Autodesk Inventor part; units mm, degrees
ref_plane "Work Plane1" through (0, 7.5, 0) normal (0, 1, 0) x (1, 0, 0)
ref_plane "YZ Plane" through (0, 0, 0) normal (1, 0, 0) x (0, 1, 0)
ref_plane "XZ Plane" through (0, 0, 0) normal (0, 1, 0) x (-1, 0, 0)
sketch "Sketch1" plane through (0, 0, 0) normal (0, 1, 0) x (-1, 0, 0)
  circle A0 centre (0, 0) radius 12.5
  dimension "d0" = 25
extrude "Extrusion1" add sketch "Sketch1" along normal blind 19 and the other way blind 15
sketch "Sketch2" plane through (0, 0, 0) normal (0, 0, 1) x (1, 0, 0)
  line L0 (-5.25, -15) -> (-5.25, -7.5)
  arc A0 (5.25, -7.5) -> (-5.25, -7.5) centre (0, -7.5) ccw
  line L1 (5.25, -7.5) -> (5.25, -15)
  line L2 (5.25, -15) -> (-5.25, -15)
  line L3 (-3.1, -15) -> (-3.1, -7.5)
  arc A1 (3.1, -7.5) -> (-3.1, -7.5) centre (0, -7.5) ccw
  line L4 (3.1, -7.5) -> (3.1, -15)
  line L5 (0, 0) -> (0, -15) construction
  line L6 (-12.5, -15) -> (12.5, -15)
  point P0 (0, -7.5)
  dimension "d5" = 10.5
  dimension "d6" = 6.2
extrude "Extrusion2" cut sketch "Sketch2" along normal mid plane 10.5
extrude "Extrusion3" cut sketch "Sketch2" against normal through all both and the other way through all contours L3 A1 L4 L2
pattern_circular "Circular Pattern1" count 2 over 90 about axis through (0, -10, 0) along (0, 1, 0) of "Extrusion2", "Extrusion3"
ref_plane "Work Plane1" through (0, 7.5, 0) normal (0, 1, 0) x (1, 0, 0)
sketch "Sketch3" plane through (0, 7.5, 0) normal (0, 1, 0) x (1, 0, 0)
  line L0 (7.2283, 10.1981) -> (6.0151, 8.9849)
  arc A0 (6.0151, 8.9849) -> (8.9849, 6.0151) centre (7.5, 7.5) ccw
  line L1 (8.9849, 6.0151) -> (10.1981, 7.2283)
  arc A1 (12.1095, 3.1) -> (3.1, 12.1095) centre (0, 0) ccw
  line L2 (0, 0) -> (7.5, 7.5) construction
  line L3 (-17.671, 0) -> (18.5127, 0)
  line L4 (5.9188, 11.0099) -> (4.9544, 10.0456)
  arc A2 (4.9544, 10.0456) -> (10.0456, 4.9544) centre (7.5, 7.5) ccw
  line L5 (10.0456, 4.9544) -> (11.0099, 5.9188)
  dimension "d15" = 4.2
  dimension "d16" = 7.5
  dimension "d17" = 45
  dimension "d18" = 7.2
extrude "Extrusion4" cut sketch "Sketch3" along normal through all both and the other way through all contours A1 L1 A0 L0
extrude "Extrusion5" cut sketch "Sketch3" against normal blind 8
pattern_circular "Circular Pattern2" count 2 over 360 about axis through (0, -10, 0) along (0, 1, 0) of "Extrusion4", "Extrusion5"
sketch "Sketch4" plane through (0, 19, 0) normal (0, 1, 0) x (1, 0, 0)
  circle A0 centre (-15.5, 15.5) radius 20.5
  line L0 (-15.5, 15.5) -> (15.5, 15.5) construction
  line L1 (15.5, 15.5) -> (15.5, -15.5) construction
  line L2 (15.5, -15.5) -> (-15.5, -15.5) construction
  line L3 (-15.5, -15.5) -> (-15.5, 15.5) construction
  circle A1 centre (-15.5, 15.5) radius 13.5
  circle A2 centre (-15.5, 15.5) radius 10.5
  point P0 (0, 0)
  point P1 (15.5, 0)
  point P2 (0, 15.5)
  dimension "d27" = 41
  dimension "d28" = 31
  dimension "d31" = 27
  dimension "d32" = 21
extrude "Extrusion6" cut sketch "Sketch4" against normal blind 8 contours A0 | A1 | A2
extrude "Extrusion7" cut sketch "Sketch4" against normal blind 12 contours A1 | A2
extrude "Extrusion8" cut sketch "Sketch4" against normal blind 16 contours A2
pattern_circular "Circular Pattern3" count 2 over 360 about axis through (0, -10, 0) along (0, 1, 0) of "Extrusion7", "Extrusion6", "Extrusion8"
properties part number "mount-stem"
Can you work these out from the model? Positions are in its coordinate system, mm. A direction names the side the tool comes from. Round coordinates to 2 decimals unless told otherwise and drop trailing zeros. Write each loop counter-clockwise with the first axis right and the second up, starting at its lowest first coordinate (ties: lowest second). Pieces come first, ordered by that corner, then holes. Notation, with made-up numbers: (11, 80) -> (19, 80) arc R22 ccw to (19, 92) -> close; hole circle Ø5 at (-1.5, 61.5). An arc over 180 degrees is marked (long way). One line per question, with ' | ' between items. Start each with the question number.
1) Suppose I cut it at C-C on x = -0.5. Write out the boundary of the cut face in (y, z).
2) I'm going to push flat-ended pins straight in: P1, Ø5, axis at y = 3.5, z = -9.5, coming from the +X side; P2, Ø8, axis at x = 8, z = 9, coming from the +Y side; P3, Ø1, axis at y = -9, z = -5, coming from the +X side. Where does each tip first touch, or does it pass through?
3) If we mould it in two halves opening along Z, with no side actions, what happens to faces 4 (the flat face through (4, 11, 4)), 5 (the cylindrical face through (6.05, -7.85, -5.98)), 6 (the cylindrical face through (-8.11, 5.03, -8.04))? For each: released by +Z, released by -Z, zero draft, split by the parting line, or undercut.
4) I need wall thicknesses on line 1 (Z direction, x = 0.5, y = -3.5); line 2 (Y direction, x = 9.5, z = -4); line 3 (X direction, y = -10.5, z = 6.75). Which ranges of each line are inside material? Lowest first, please. Write a range as [from, to].
5) Suppose I cut it at A-A on y = -9.5. Write out the boundary of the cut face in (x, z).
6) On a 3-axis mill with a long thin cutter (end or side, diameter ignored), from which of +Z, -Z, +X, -X, +Y, -Y can I reach the whole of each face in a straight line? I mean faces 1 (the flat face through (5.8, -0.5, -5.9)), 2 (the cylindrical face through (-3.8, -2.25, 0.04)), 3 (the flat face through (6.63, 13.17, -9.6)). Say none if no direction works.
7) Suppose I cut it at D-D on y = 0. Write out the boundary of the cut face in (x, z).
Return value:
1) outline: (-4.44, -12.49) -> (11, -12.49) -> (11, -1.53) -> (19, -1.53) -> (19, 2.68) -> (11, 2.68) -> (11, 12.49) -> (-4.44, 12.49) -> (-4.44, 5.25) -> (-2.27, 5.25) -> (-2.27, 0.5) arc R5.25 cw to (-2.27, -0.5) -> (-2.27, -5.25) -> (-4.44, -5.25) -> close
2) P1: stops at x = 5.92 | P2: stops at y = 11 | P3: stops at x = 11.66
3) face 4: zero draft | face 5: undercut | face 6: released by -Z
4) line 1: z = [-12.49, -5.25], [5.25, 12.49] | line 2: y = [-15, 11] | line 3: x = [-10.52, -9.72], [-5.54, -3.1], [3.1, 10.52]
5) outline: (-12.11, -3.1) arc R12.5 ccw to (-3.1, -12.11) -> (-3.1, -5.25) -> (-5.25, -5.25) -> (-5.25, -3.1) -> close; (-12.11, 3.1) -> (-5.25, 3.1) -> (-5.25, 5.25) -> (-3.1, 5.25) -> (-3.1, 12.11) arc R12.5 ccw to (-7.23, 10.2) -> (-6.02, 8.98) arc R2.1 cw to (-8.98, 6.02) -> (-10.2, 7.23) arc R12.5 ccw to start; (3.1, -12.11) arc R12.5 ccw to (7.23, -10.2) -> (6.02, -8.98) arc R2.1 cw to (8.98, -6.02) -> (10.2, -7.23) arc R12.5 ccw to (12.11, -3.1) -> (5.25, -3.1) -> (5.25, -5.25) -> (3.1, -5.25) -> close; (3.1, 5.25) -> (5.25, 5.25) -> (5.25, 3.1) -> (12.11, 3.1) arc R12.5 ccw to (3.1, 12.11) -> close
6) face 1: none | face 2: -Y | face 3: +X, +Y, -Y
7) outline: (-11.01, 5.92) arc R12.5 ccw to (5.92, -11.01) -> (4.95, -10.05) arc R3.6 cw to (10.05, -4.95) -> (11.01, -5.92) arc R12.5 ccw to (-5.92, 11.01) -> (-4.95, 10.05) arc R3.6 cw to (-10.05, 4.95) -> close
